Geometry: see drawing. Coordinates: mm, zero at the bounding-box minimum. A direction names the side the tool comes from. Coordinates: 2 decimals unless noted, no trailing zeros. Order: outer loops, then holes, each group sorted by start corner. A loop starts at its lowest first (then second) coordinate and runs counter-clockwise, first axis right, second up. Notation, with made-up numbers: (76.5, -40) -> (132.5, -40) arc R6 ccw to (132.5, -33) -> close; hole circle Ø10 at (46, -21). An arc over 180 degrees is marked (long way). One line per item, written item: value. Start each with the question number.
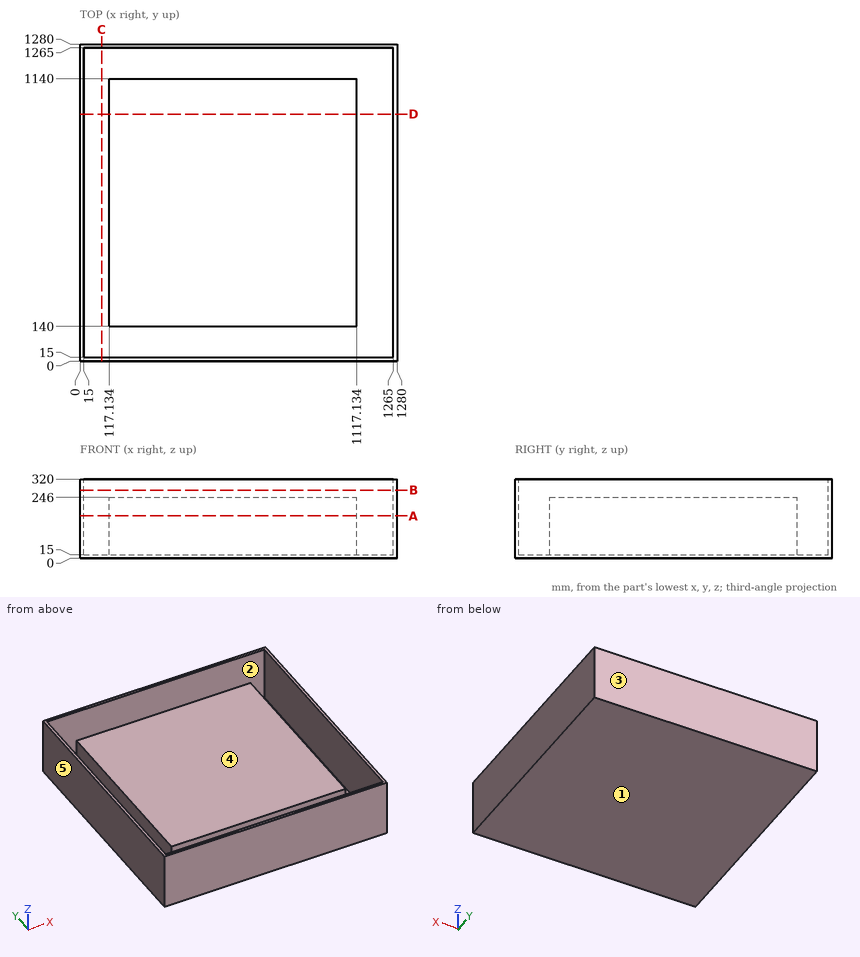
1) Mould query, pull axis X, two halves, no side actions, for the marked faces 3, 4 and 5. Classes: +X half, -X half, draft (parallel to the pull), parting line (faces both ways), or undercut.
2) Ray query, line 1 along Y through (x, z) = (1107.5, 158.5); line 2 along X through (y, z) = (170, 177.5); line 3 along X through (y, z) = (690, 273). Return the intervals inside material, ascending. Write a range as from..to.
3) Access query for the marked faces 1 and 2. Directions: +Z, -Z, +X, -X, +Y, -Y. A direction counts if a zero-diameter tool reaches every point of the face in a straight line with its end or side. Return the directions, or none.
4) Section query D-D, the plane y = 996.5. Return the cut outline in (x, z).
5) Section query A-A, the plane z = 171.5. Return the cut outline in (x, y).
6) Section query B-B, the plane z = 275.5. Return the cut outline in (x, y).
7) Section query C-C, the plane x = 87. Return the cut outline in (y, z), plus the area to 4 significant figures.
Entries:
1. face 3: draft
1. face 4: undercut
1. face 5: -X half
2. line 1: y = 0..15, 140..1140, 1265..1280
2. line 2: x = 0..15, 117.13..1117.13, 1265..1280
2. line 3: x = 0..15, 1265..1280
3. face 1: -Z, +X, -X, +Y, -Y
3. face 2: +Z
4. outline: (0, 0) -> (1280, 0) -> (1280, 320) -> (1265, 320) -> (1265, 15) -> (1117.13, 15) -> (1117.13, 246) -> (117.13, 246) -> (117.13, 15) -> (15, 15) -> (15, 320) -> (0, 320) -> close
5. outline: (0, 0) -> (1280, 0) -> (1280, 1280) -> (0, 1280) -> close; (117.13, 140) -> (1117.13, 140) -> (1117.13, 1140) -> (117.13, 1140) -> close; hole (15, 15) -> (1265, 15) -> (1265, 1265) -> (15, 1265) -> close
6. outline: (0, 0) -> (1280, 0) -> (1280, 1280) -> (0, 1280) -> close; hole (15, 15) -> (1265, 15) -> (1265, 1265) -> (15, 1265) -> close
7. outline: (0, 0) -> (1280, 0) -> (1280, 320) -> (1265, 320) -> (1265, 15) -> (15, 15) -> (15, 320) -> (0, 320) -> close
7. area: 28,350 mm2
